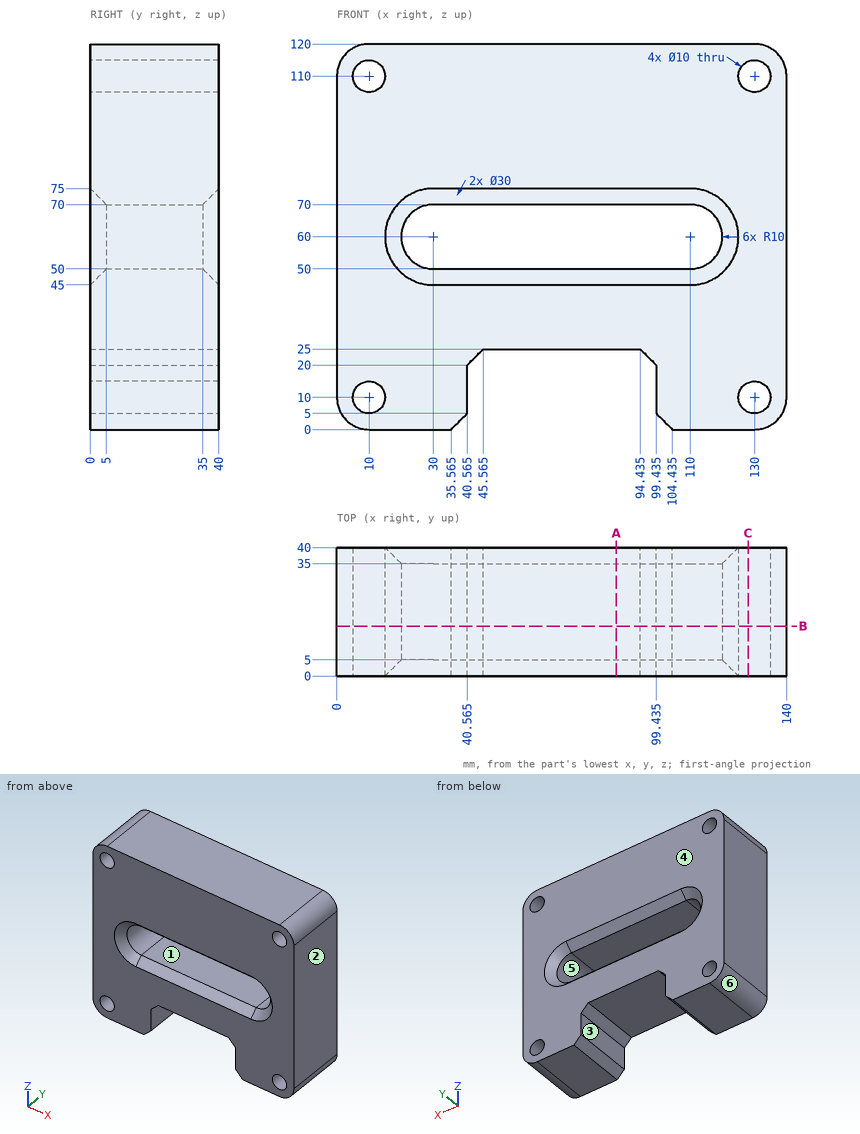
Print and shaded views of the part. All mm, measured from the part's lowest x, y and z. A direction names the side the tool comes from. Give positions to 0.01 mm unless a question says otherwise; leave off trailing zeros. Loops run counter-clockwise (first coordinate to the right, second up) from the corner with the lowest first, then second, coordinate; pieces in that order, holes last. Notation, with made-up numbers: (75.5, 84.25) - (98.5, 84.25) arc R18 cw to (98.5, 106.25) - close; hole circle Ø1 at (36.5, 44). An arc over 180 degrees is marked (long way). Use a Markdown table: item, result.
(1) Drop flat-ended pins along their axis: pin 1 Ø12 at (x, y) = (85, 23.5) entering from -Z; pin 2 Ø9 at (x, z) = (10, 10) entering from +Y; pin 3 Ø11.5 at (x, z) = (130, 10) entering from -Y; pin 4 Ø10 at (x, z) = (25, 54.5) entering from -Y. Give the stop position or say it passes through.
Taken from the geometry:
| item | result |
|---|---|
| pin 1 | z = 25 |
| pin 2 | through |
| pin 3 | y = 0 |
| pin 4 | y = 2.57 |
(2) Band-saw the part on C-C (x = 128). Give the cut face in (y, z), and give its area (3 significant figures).
Taken from the geometry:
| item | result |
|---|---|
| outline | (0, 0) - (40, 0) - (40, 5.42) - (0, 5.42) - close; (0, 14.58) - (40, 14.58) - (40, 105.42) - (0, 105.42) - close; (0, 114.58) - (40, 114.58) - (40, 120) - (0, 120) - close |
| area | 4,070 mm2 |
(3) Pull direction Z, two halves, no side cores. Call the marked faces 4, 5 and 6: +Z half, -Z half, draft (parallel to the pull), parting line (faces both ways), or undercut.
Taken from the geometry:
| item | result |
|---|---|
| face 4 | draft |
| face 5 | undercut |
| face 6 | -Z half |
(4) Which spindle directions (+Z, -Z, +X, -X, +Y, -Y) get a long thin tool onto all of the face, cutting with end or side? Do the marked faces 1, 2 and 3. Say none if no direction does.
Taken from the geometry:
| item | result |
|---|---|
| face 1 | +Y, -Y |
| face 2 | +Z, -Z, +X, +Y, -Y |
| face 3 | -Z, +Y, -Y |
(5) Band-saw the part on A-A (x = 87). Give the cut face in (y, z).
Taken from the geometry:
| item | result |
|---|---|
| outline | (0, 25) - (40, 25) - (40, 45) - (35, 50) - (5, 50) - (0, 45) - close; (0, 75) - (5, 70) - (35, 70) - (40, 75) - (40, 120) - (0, 120) - close |
(6) Band-saw the part on B-B (y = 15.5). Give the cut face in (x, z) (1 decimal), and give its area (3 significant figures).
Taken from the geometry:
| item | result |
|---|---|
| outline | (0, 10) arc R10 ccw to (10, 0) - (35.6, 0) - (40.6, 5) - (40.6, 20) - (45.6, 25) - (94.4, 25) - (99.4, 20) - (99.4, 5) - (104.4, 0) - (130, 0) arc R10 ccw to (140, 10) - (140, 110) arc R10 ccw to (130, 120) - (10, 120) arc R10 ccw to (0, 110) - close; hole circle Ø10 at (10, 10); hole circle Ø10 at (10, 110); hole (30, 50) - (110, 50) arc R10 ccw to (110, 70) - (30, 70) arc R10 ccw to start; hole circle Ø10 at (130, 10); hole circle Ø10 at (130, 110) |
| area | 13,000 mm2 |
(7) Wall check: line 1 along X through (y, z) = (31.5, 10) (1 decimal); line 2 along X through (y, z) = (31, 110); line 3 along Z through (x, y) = (10, 14). Give the ranges that are in metal, low to high.
Taken from the geometry:
| item | result |
|---|---|
| line 1 | 0 to 5, 15 to 40.6, 99.4 to 125, 135 to 140 |
| line 2 | 0 to 5, 15 to 125, 135 to 140 |
| line 3 | 0 to 5, 15 to 105, 115 to 120 |
